The model under review builds one solid part; all positions refer to its coordinate system, in mm. Face numbers are marked on the shaded views. A direction names the side the tool comes from. Round coordinates to 2 decimals unless told otherwise and drop trailing zeros. Write each loop counter-clockwise with the first axis right and the second up, starting at its lowest first coordinate (ties: lowest second). Pieces come first, ordered by that corner, then holes. Notation, with made-up numbers: M 80,18 L 111,18 A28 ccw 111,39 Z; hole C 80,-17.5 d10. An arc over 180 degrees is marked long. One line per item, written item: value. Start each with the question number.
1) Take a section at B-B, the plane x = 122. Write out the cut boundary in (y, z), and give its area (3 significant figures).
2) Take a section at A-A, the plane z = 40. Write out the cut boundary in (x, y).
3) Take a section at C-C, the plane z = 10. Write out the cut boundary in (x, y), and give its area (3 significant figures).
4) For P1, Ø12, axis at y = -1.5, z = 16.5, coming from the -X side; P2, Ø6, axis at y = -21.5, z = 32, coming from the +X side; P3, Ø4, axis at y = -21, z = 43, coming from the -X side, all flat-tipped, find the tip position at first contact; note any pin that passes through.
5) Tool access review of the marked faces 5 and 6: name each direction out of +Z, -Z, +X, -X, +Y, -Y from which nothing blocks a thin tool from reaching the whole face with its end or side.
6) Wall thickness on probe 1 along Y at (x, z) = (27.5, 4); probe 2 along X at (y, z) = (-0.5, 60); probe 3 along Z at (x, y) = (118.5, -42): over which ranges is each line inside the solid? List them lowest first.
7) Take a section at D-D, the plane y = 0. State how many separate pieces and enclosed holes the cut face has, and give its area (3 significant figures).
8) Mouldability with a two-part tool opening along Y and no side actions: class the marked faces 1, 2, 3 and 4 as +Y half, -Y half, draft (parallel to the pull), parting line (faces both ways), or undercut.
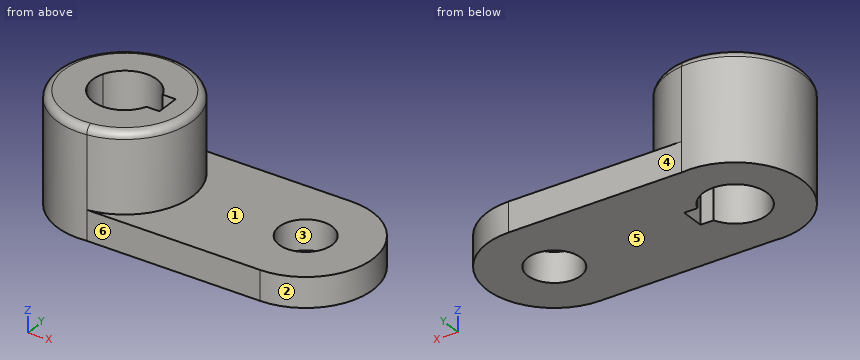
from build123d import *

# Parameters (mm, degrees)
F0_R     = 41.7429221606
F1_DEPTH = 75.438
F0_R_2   = 18.342139753
F2_DEPTH = 20.574
F3_DEPTH = 73
F4_R     = 5


with BuildPart() as f1:
    # F0 (on Top) → F1 (new body)
    with BuildSketch(Plane.XY):
        with BuildLine():
            ThreePointArc((5.3434108118, -46.5023219585), (34.9366141904, -31.1520621396), (46.8083110851, 0))
            ThreePointArc((46.8083110851, 0), (34.9366141904, 31.1520621396), (5.3434108118, 46.5023219585))
            ThreePointArc((5.3434108118, 46.5023219585), (-46.8083110851, 0), (5.3434108118, -46.5023219585))
        make_face()
        Circle(F0_R, mode=Mode.SUBTRACT)
        Circle(F0_R)
        with BuildLine():
            ThreePointArc((-20.5937367847, -8.2344636321), (-22.1790077791, 0), (-20.5937367847, 8.2344636321))
            ThreePointArc((-20.5937367847, 8.2344636321), (0, 22.1790077791), (20.5937367847, 8.2344636321))
            Line((20.5937367847, 8.2344636321), (29.5797027647, 8.2344636321))
            Line((29.5797027647, 8.2344636321), (29.5797027647, -8.2344636321))
            Line((29.5797027647, -8.2344636321), (20.5937367847, -8.2344636321))
            ThreePointArc((20.5937367847, -8.2344636321), (0, -22.1790077791), (-20.5937367847, -8.2344636321))
        make_face(mode=Mode.SUBTRACT)
    extrude(amount=F1_DEPTH)

    # F0 (on Top) → F2 (join)
    with BuildSketch(Plane.XY):
        with BuildLine():
            ThreePointArc((5.3434108118, 46.5023219585), (34.9366141904, 31.1520621396), (46.8083110851, 0))
            ThreePointArc((46.8083110851, 0), (34.9366141904, -31.1520621396), (5.3434108118, -46.5023219585))
            Line((5.3434108118, -46.5023219585), (125.1767128706, -46.5023219585))
            ThreePointArc((125.1767128706, -46.5023219585), (171.6790348291, 0), (125.1767128706, 46.5023219585))
            Line((125.1767128706, 46.5023219585), (5.3434108118, 46.5023219585))
        make_face()
        with Locations((125.1767128706, 0)):
            Circle(F0_R_2, mode=Mode.SUBTRACT)
    extrude(amount=F2_DEPTH)

    # F0 (on Top) → F3 (join)
    with BuildSketch(Plane.XY):
        with BuildLine():
            ThreePointArc((5.3434108118, -46.5023219585), (34.9366141904, -31.1520621396), (46.8083110851, 0))
            ThreePointArc((46.8083110851, 0), (34.9366141904, 31.1520621396), (5.3434108118, 46.5023219585))
            ThreePointArc((5.3434108118, 46.5023219585), (-46.8083110851, 0), (5.3434108118, -46.5023219585))
        make_face()
        Circle(F0_R, mode=Mode.SUBTRACT)
    extrude(amount=F3_DEPTH)

    # F4
    f4_edges = [f1.edges().sort_by_distance(p)[0] for p in [
        (-5.343411, 46.502322, 75.438),
    ]]
    fillet(f4_edges, radius=F4_R)


solid = f1.part
Checked values:
1. outline: M -46.5,0 L -18.06,0 L -18.06,20.57 L -46.5,20.57 Z; M 18.06,0 L 46.5,0 L 46.5,20.57 L 18.06,20.57 Z
1. area: 1,170 mm2
2. outline: C 0,0 d93.62; hole M 20.59,-8.23 L 29.58,-8.23 L 29.58,8.23 L 20.59,8.23 A22.18 ccw long Z
3. outline: M 5.34,-46.5 L 125.18,-46.5 A46.5 ccw 125.18,46.5 L 5.34,46.5 A46.81 ccw long Z; hole M 20.59,-8.23 L 29.58,-8.23 L 29.58,8.23 L 20.59,8.23 A22.18 ccw long Z; hole C 125.18,0 d36.68
3. area: 15,700 mm2
4. P1: stops at x = -46.81
4. P2: stops at x = 43
4. P3: stops at x = -42.78
5. face 5: -Z, +X, -X, +Y, -Y
5. face 6: +Z, -Z, +X, -Y
6. probe 1: y = -46.5 to -8.23, 8.23 to 46.5
6. probe 2: x = -46.81 to -22.17, 29.58 to 46.81
6. probe 3: z = 0 to 20.57
7. separate pieces: 3
7. enclosed holes: 0
7. area: 4,960 mm2
8. face 1: draft
8. face 2: parting line
8. face 3: undercut
8. face 4: +Y half
